```python
from build123d import *

# Parameters (mm, degrees)
CROQUIS1_W              = 200
CROQUIS1_H              = 200
CROQUIS1_R              = 2.5
CROQUIS1_W_2            = 158
CROQUIS1_H_2            = 158
SALIENTE_EXTRUIR1_DEPTH = 40


with BuildPart() as part:
    # Croquis1 → Saliente-Extruir1 (new body)
    with BuildSketch(Plane(origin=(0, 0, 0), x_dir=(1, 0, 0), z_dir=(0, 1, 0))):
        with Locations((100, 100)):
            Rectangle(CROQUIS1_W, CROQUIS1_H)
        with Locations(Location((185, 185, 0), (0, 0, 270))):
            Circle(CROQUIS1_R, mode=Mode.SUBTRACT)
        with Locations(Location((185, 15, 0), (0, 0, 270))):
            Circle(CROQUIS1_R, mode=Mode.SUBTRACT)
        with Locations(Location((15, 15, 0), (0, 0, 270))):
            Circle(CROQUIS1_R, mode=Mode.SUBTRACT)
        with Locations(Location((15, 185, 0), (0, 0, 270))):
            Circle(CROQUIS1_R, mode=Mode.SUBTRACT)
        with Locations((100, 100)):
            Rectangle(CROQUIS1_W_2, CROQUIS1_H_2, mode=Mode.SUBTRACT)
    extrude(amount=SALIENTE_EXTRUIR1_DEPTH)


solid = part.part
```
Work out the finished part from the listing and answer in its coordinate system (mm). A direction names the side the tool comes from. Give positions to 0.01 mm unless a question says otherwise; leave off trailing zeros. Loops run counter-clockwise (first coordinate to the right, second up) from the corner with the lowest first, then second, coordinate; pieces in that order, holes last. Notation, with made-up numbers: (54.25, 72.25) -> (106.25, 72.25) arc R15 cw to (106.25, 78.25) -> close; hole circle Ø9 at (-16, 36.25). An arc over 180 degrees is marked (long way). Put each result on its own line as item: value. Start each with the question number.
Item 1: The part is cut by section B-B (x = 185). Give the vertices of the cut face in (y, z).
Item 2: Find the intervals of material crossed by L1, parallel to X at y = 8, z = -15; L2, parallel to Z at x = 185, y = 22; L3, parallel to X at y = 21.5, z = -32.5, in increasing order. Write a range as [from, to].
Item 3: Which of the six approach directions +Z, -Z, +X, -X, +Y, -Y give full straight-line access (tool end or side, diameter ignored) to faces 1 (the face through (99, 20, -179)), 2 (the face through (0, 20, -99))?
Item 4: The part is cut by section A-A (z = -185). Give the vertices of the cut face in (x, y).
Item 5: The part is cut by section C-C (x = 45.5). Give the vertices of the cut face in (y, z).
Item 6: This flat-tipped pin is pushed along its axis until it touches: P1, Ø1, axis at x = 177, z = -22.5, coming from the +Y side. Where does it stop, or does it pass through?
Item 7: The part is cut by section D-D (z = -157.5). Give the vertices of the cut face in (x, y).
Answers below:
1. outline: (0, -200) -> (40, -200) -> (40, -187.5) -> (0, -187.5) -> close; (0, -182.5) -> (40, -182.5) -> (40, -17.5) -> (0, -17.5) -> close; (0, -12.5) -> (40, -12.5) -> (40, 0) -> (0, 0) -> close
2. L1: [0, 12.5], [17.5, 182.5], [187.5, 200]
2. L2: [-200, -187.5], [-182.5, -17.5], [-12.5, 0]
2. L3: [0, 21], [179, 200]
3. face 1: +Y, -Y
3. face 2: +Z, -Z, -X, +Y, -Y
4. outline: (0, 0) -> (12.5, 0) -> (12.5, 40) -> (0, 40) -> close; (17.5, 0) -> (182.5, 0) -> (182.5, 40) -> (17.5, 40) -> close; (187.5, 0) -> (200, 0) -> (200, 40) -> (187.5, 40) -> close
5. outline: (0, -200) -> (40, -200) -> (40, -179) -> (0, -179) -> close; (0, -21) -> (40, -21) -> (40, 0) -> (0, 0) -> close
6. P1: through
7. outline: (0, 0) -> (21, 0) -> (21, 40) -> (0, 40) -> close; (179, 0) -> (200, 0) -> (200, 40) -> (179, 40) -> close
